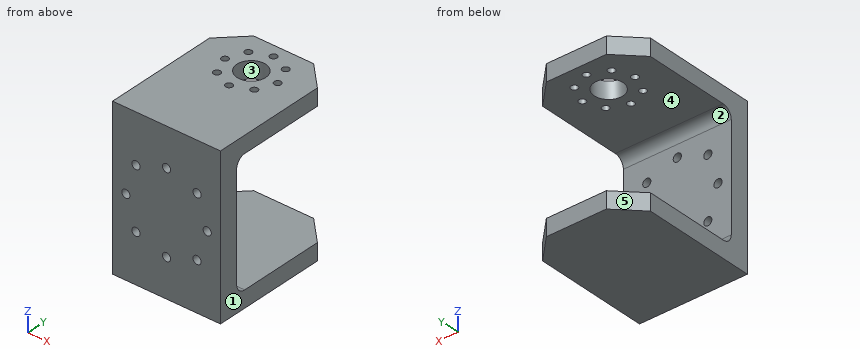
Autodesk Inventor part; units mm, degrees
ref_plane "YZ Plane" through (0, 0, 0) normal (1, 0, 0) x (0, 1, 0)
ref_plane "XZ Plane" through (0, 0, 0) normal (0, 1, 0) x (-1, 0, 0)
ref_plane "XY Plane" through (0, 0, 0) normal (0, 0, 1) x (1, 0, 0)
sketch "Skizze1" plane through (0, 0, 0) normal (0, 1, 0) x (-1, 0, 0)
  line L0 (-22.5, 33) -> (22.5, 33)
  line L1 (22.5, 33) -> (22.5, -33)
  line L2 (22.5, -33) -> (-22.5, -33)
  line L3 (-22.5, -33) -> (-22.5, 33)
  line L4 (-22.5, 33) -> (22.5, -33) construction
  line L5 (22.5, 33) -> (-22.5, -33) construction
  point P0 (0, 0)
  dimension "d0" = 45
  dimension "d1" = 66
extrude "Extrusion1" add sketch "Skizze1" along normal blind 8
sketch "Skizze2" plane through (0, 8, 0) normal (0, 1, 0) x (1, 0, 0)
  line L0 (-22.5, -33) -> (22.5, -33)
  line L1 (22.5, -33) -> (22.5, 33)
  line L2 (22.5, 33) -> (-22.5, 33)
  line L3 (-22.5, 33) -> (-22.5, -33)
  line L4 (-22.5, -33) -> (22.5, -33)
  line L5 (22.5, -33) -> (22.5, -26)
  line L6 (22.5, -26) -> (-22.5, -26)
  line L7 (-22.5, -26) -> (-22.5, -33)
  line L8 (22.5, 33) -> (-22.5, 33)
  line L9 (-22.5, 33) -> (-22.5, 26)
  line L10 (-22.5, 26) -> (22.5, 26)
  line L11 (22.5, 26) -> (22.5, 33)
  point P0 (0, 0)
  dimension "d4" = 7
  dimension "d5" = 7
extrude "Extrusion2" add sketch "Skizze2" along normal blind 50 contours L3 L6 L1 L0 | L3 L2 L1 L10
sketch "Skizze3" plane through (0, 8, 0) normal (0, 1, 0) x (1, 0, 0)
  line L0 (-22.5, -26) -> (22.5, -26) construction
  line L1 (22.5, -26) -> (22.5, 26) construction
  line L2 (22.5, 26) -> (-22.5, 26) construction
  line L3 (-22.5, 26) -> (-22.5, -26) construction
  line L4 (-22.5, -26) -> (22.5, 26) construction
  line L5 (-22.5, 26) -> (22.5, 26) construction
  line L6 (22.5, -26) -> (-22.5, 26) construction
  line L7 (16.9706, 0) -> (0, 16.9706) construction
  line L8 (0, 16.9706) -> (-16.9706, 0) construction
  line L9 (-16.9706, 0) -> (0, -16.9706) construction
  line L10 (0, -16.9706) -> (16.9706, 0) construction
  line L11 (16.9706, 0) -> (-16.9706, 0) construction
  line L12 (0, 16.9706) -> (0, -16.9706) construction
  circle A0 centre (0, 0) radius 18 construction
  line L13 (17.4913, 17.4913) -> (-17.5019, -17.5019) construction
  line L14 (16.4193, -16.4193) -> (-16.3603, 16.3603) construction
  point P0 (0, 0)
  point P1 (0, 0)
  point P2 (-12.7279, -12.7279)
  point P3 (12.7279, -12.7279)
  point P4 (12.7279, 12.7279)
  point P5 (-12.7279, 12.7279)
  dimension "d12" = 24
  dimension "d13" = 24
  dimension "d14" = 36
hole "Bohrung1" at (-16.9706, 8, 0) at (0, 8, -16.9706) at (16.9706, 8, 0) at (0, 8, 16.9706) at (-12.7279, 8, 12.7279) at (-12.7279, 8, -12.7279) at (12.7279, 8, -12.7279) at (12.7279, 8, 12.7279) direction (0, -1, 0) diameter 3.4 end through all
sketch "Skizze4" plane through (-22.5, 0, 33) normal (0, 0, 1) x (1, 0, 0)
  line L0 (22.5, 0) -> (22.5, 74.8441) construction
  line L1 (0, 58) -> (45, 58)
  circle A0 centre (22.5, 42) radius 6
  line L2 (45, 0) -> (45, 52)
  line L3 (0, 52) -> (45, 52)
  line L4 (0, 0) -> (0, 52)
  point P0 (22.5, 53)
  dimension "d22" = 5
  dimension "d23" = 11
  dimension "d34" = 12
hole "Bohrung2" at (0, 53, 33) direction (0, 0, -1) diameter 2.9 end up to surface
pattern_circular "Runde Anordnung1" count 8 over 360 about axis through (0, 42, 33) along (0, 0, 1) of "Bohrung2"
extrude "Extrusion3" cut sketch "Skizze4" against normal up to surface (7 mm away)
chamfer "Fase1" distance 10 angle 45 4 edges at (-22.5, 58, 29.5) (-22.5, 58, -29.5) (22.5, 58, 29.5) (22.5, 58, -29.5)
fillet "Rundung1" radius 4 2 edges at (0, 8, 26) (0, 8, -26)
equation "\"d4\" = d5"
properties part number "frame_mx108" material "Aluminium 6061"
Build history of the part. All positions in model axes, mm. Face numbers are marked on the shaded views. A direction names the side the tool comes from. Round coordinates to 2 decimals unless told otherwise and drop trailing zeros. Loops run counter-clockwise (first coordinate to the right, second up) from the corner with the lowest first, then second, coordinate; pieces in that order, holes last. Notation, with made-up numbers: (70, -32) -> (74, -32) arc R23 ccw to (74, -11) -> close; hole circle Ø10 at (-38.5, 83.25). An arc over 180 degrees is marked (long way). One line per item, written item: value. Start each with the question number.
Q1. Two-plate mould, pull along X, no slides. Class the marked faces 1, 2 and 3: released by +X, released by -X, zero draft, split by the parting line, or undercut.
Q2. Cut at A-A on y = 31. List the corners of the cut face in (x, z), plus the area to 3 significant figures.
Q3. Drop flat-ended pins along their axis: pin 1 Ø1.5 at (x, z) = (-2, 10) entering from +Y; pin 2 Ø2.5 at (x, z) = (-12.73, 12.73) entering from +Y. Give the stop position or say it passes through.
Q4. 3-axis set-ups, long thin cutter, end or side, ignore diameter. For the marked faces 4 and 5: which of +Z, -Z, +X, -X, +Y, -Y reach the whole face in a straight line?
Q5. Cut at C-C on z = 0. List the corners of the cut face in (x, y), plus the area to 3 significant figures.
Q6. Probe line 1 along X through (y, z) = (4.5, 0); line 2 along Z through (x, y) = (0, 4.5); line 3 along Y through (x, z) = (0, 29.75). List the from-to ranges inside material, lowest first.
Q7. Cut at D-D on x = 5. List the corners of the cut face in (y, z), plus the area to 3 significant figures.
Q8. Cut at B-B on x = 0. Count the separate pieces of the cut face and the enclosed holes in it, plus the area to 3 significant figures.
Computed:
1. face 1: released by +X
1. face 2: zero draft
1. face 3: undercut
2. outline: (-22.5, -33) -> (22.5, -33) -> (22.5, -26) -> (-22.5, -26) -> close; (-22.5, 26) -> (-1.45, 26) -> (-1.45, 33) -> (-22.5, 33) -> close; (1.45, 26) -> (22.5, 26) -> (22.5, 33) -> (1.45, 33) -> close
2. area: 610 mm²
3. pin 1: y = 8
3. pin 2: through
4. face 4: +X, -X, +Y
4. face 5: +Z, -Z, -X, +Y
5. outline: (-22.5, 0) -> (-18.67, 0) -> (-18.67, 8) -> (-22.5, 8) -> close; (-15.27, 0) -> (15.27, 0) -> (15.27, 8) -> (-15.27, 8) -> close; (18.67, 0) -> (22.5, 0) -> (22.5, 8) -> (18.67, 8) -> close
5. area: 306 mm²
6. line 1: -22.5 to -18.67, -15.27 to 15.27, 18.67 to 22.5
6. line 2: -33 to -18.67, -15.27 to 15.27, 18.67 to 33
6. line 3: 0 to 29.55, 32.45 to 36, 48 to 51.55, 54.45 to 58
7. outline: (0, -33) -> (58, -33) -> (58, -26) -> (12, -26) arc R4 cw to (8, -22) -> (8, 22) arc R4 cw to (12, 26) -> (38.68, 26) -> (38.68, 33) -> (0, 33) -> close; (45.32, 26) -> (58, 26) -> (58, 33) -> (45.32, 33) -> close
7. area: 1,190 mm²
8. separate pieces: 6
8. enclosed holes: 0
8. area: 1,060 mm²
